from build123d import *


with BuildPart() as part:
    # Schizzo1 → Rivoluzione1 (revolve)
    with BuildSketch(Plane.XY):
        with BuildLine():
            Line((0, 0), (-26, 0))
            ThreePointArc((-26, 0), (-29.535533906, 1.464466094), (-31, 5))
            Line((-31, 5), (-31, 110))
            Line((-31, 110), (-13, 211))
            Line((-13, 211), (-13, 225))
            Line((-13, 225), (-8.5, 225))
            Line((-8.5, 225), (-8.5, 220.5))
            Line((-8.5, 220.5), (-8.5, 210.602144339))
            Line((-8.5, 210.602144339), (-26.5, 109.602144339))
            Line((-26.5, 109.602144339), (-26.5, 5))
            ThreePointArc((-26.5, 5), (-26.353553391, 4.646446609), (-26, 4.5))
            Line((-26, 4.5), (-4.5, 4.5))
            Line((-4.5, 4.5), (0, 4.5))
            Line((0, 4.5), (0, 0))
        make_face()
    revolve(axis=Axis((0, 225, 0), (0, -1, 0)))


solid = part.part
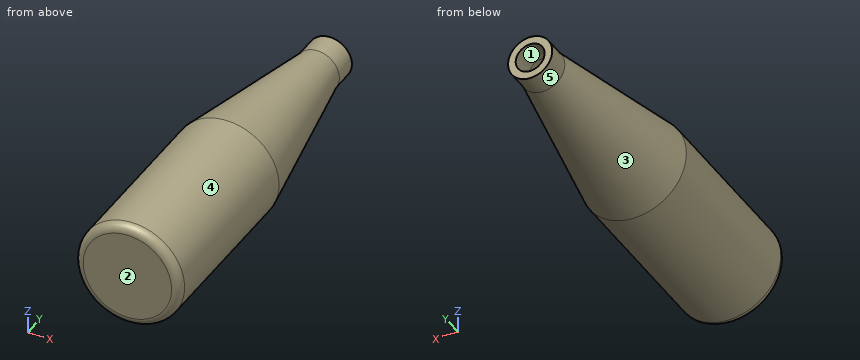
Source: CAD feature listing. Evaluate the final solid. Frame: model axes, mm. Face numbers are marked on the shaded views. A direction names the side the tool comes from. Give positions to 0.01 mm unless a question says otherwise; leave off trailing zeros. Write each loop counter-clockwise with the first axis right and the second up, starting at its lowest first coordinate (ties: lowest second). Pieces come first, ordered by that corner, then holes. Notation, with made-up numbers: (62.25, -4) - (81.25, -4) arc R12 cw to (81.25, 18) - close; hole circle Ø2 at (89, 43). An arc over 180 degrees is marked (long way). Write item = value, one per line. Start each with the question number.
Q1. Reachability of the marked faces 4 and 5 from +Z, -Z, +X, -X, +Y, -Y: full face, straight path, thin tool, end or side. Return the list, or none.
Q2. Cut plane B-B, the plane y = 84. Return loops of the section in (x, z).
Q3. Cut plane D-D, the plane y = 116.5. Return loops of the section in (x, z), then the cut area to 3 significant figures.
Q4. Material intervals for probe 1 along X at (y, z) = (217.75, 0); probe 2 along X at (y, z) = (86, 0), sorted ascending.
Q5. Cut plane A-A, the plane z = 0. Return loops of the section in (x, y), then the cut area to 3 significant figures.
Q6. Draft query along X for the marked faces 1, 2 and 3. Return one class per face: +X half, -X half, draft (parallel to the pull), parting line (faces both ways), or undercut.
Q7. Pin query (flat end, axial travel): pin 1 Ø1 at (y, z) = (151.5, 3) entering from -X; pin 2 Ø13.5 at (x, z) = (0, 0) entering from +Y; pin 3 Ø5 at (x, y) = (-21, 122.5) entering from +Z. Return the tip coordinate at first contact, or that it passes through.
Q8. Cut plane C-C, the plane x = 0. Return loops of the section in (y, z).
Computed values:
q1.face_4 = +Y, -Y
q1.face_5 = +Y
q2.outline = circle Ø62 at (0, 0); hole circle Ø53 at (0, 0)
q3.outline = circle Ø59.68 at (0, 0); hole circle Ø50.54 at (0, 0)
q3.area = 791 mm²
q4.probe_1 = -13 to -8.5, 8.5 to 13
q4.probe_2 = -31 to -26.5, 26.5 to 31
q5.outline = (-31, 5) arc R5 ccw to (-26, 0) - (26, 0) arc R5 ccw to (31, 5) - (31, 110) - (13, 211) - (13, 225) - (8.5, 225) - (8.5, 210.6) - (26.5, 109.6) - (26.5, 5) arc R0.5 cw to (26, 4.5) - (-26, 4.5) arc R0.5 cw to (-26.5, 5) - (-26.5, 109.6) - (-8.5, 210.6) - (-8.5, 225) - (-13, 225) - (-13, 211) - (-31, 110) - close
q5.area = 2,270 mm²
q6.face_1 = undercut
q6.face_2 = draft
q6.face_3 = parting line
q7.pin_1 = -23.52
q7.pin_2 = 4.5
q7.pin_3 = 22.12
q8.outline = (0, -26) arc R5 ccw to (5, -31) - (110, -31) - (211, -13) - (225, -13) - (225, -8.5) - (210.6, -8.5) - (109.6, -26.5) - (5, -26.5) arc R0.5 cw to (4.5, -26) - (4.5, 26) arc R0.5 cw to (5, 26.5) - (109.6, 26.5) - (210.6, 8.5) - (225, 8.5) - (225, 13) - (211, 13) - (110, 31) - (5, 31) arc R5 ccw to (0, 26) - close
